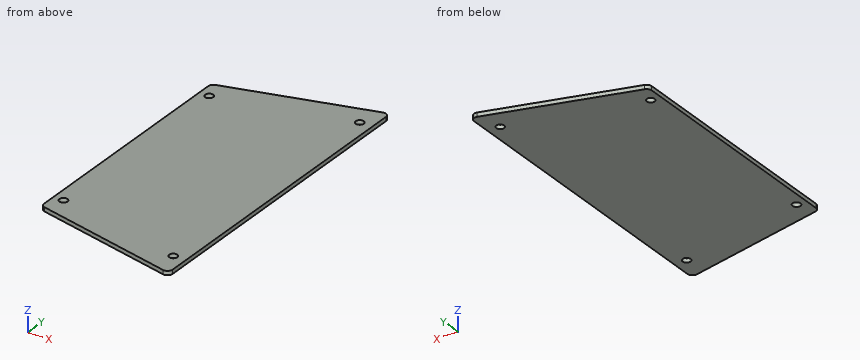
Autodesk Inventor part; units mm, degrees
ref_plane "YZ Plane" through (0, 0, 0) normal (1, 0, 0) x (0, 1, 0)
ref_plane "XZ Plane" through (0, 0, 0) normal (0, 1, 0) x (-1, 0, 0)
ref_plane "XY Plane" through (0, 0, 0) normal (0, 0, 1) x (1, 0, 0)
sketch "Esquisse1" plane through (0, 0, 0) normal (0, 0, 1) x (1, 0, 0)
  line L0 (0, 0) -> (60, 0)
  line L1 (60, 0) -> (60, 130)
  line L2 (60, 130) -> (0, 130)
  line L3 (0, 130) -> (0, 0)
  dimension "d0" = 130
  dimension "d1" = 60
extrude "Extrusion1" add sketch "Esquisse1" along normal blind 1.6
chamfer "Chanfrein1" distance 58 distance2 15 1 edges at (0, 130, 0.8) measured on face at (40, 130, 0.5333)
chamfer "Chanfrein2" distance 15 distance2 58 1 edges at (0, 0, 0.8) measured on face at (0, 76.6667, 1.0667)
fillet "Congé1" radius 2 6 edges at (60, 0, 0.8) (0, 15, 0.8) (0, 115, 0.8) (60, 130, 0.8) (58, 130, 0.8) (58, 0, 0.8)
sketch "Esquisse2" plane through (0, 0, 1.6) normal (0, 0, 1) x (1, 0, 0)
  circle A0 centre (4, 22) radius 1.6
  circle A1 centre (55, 10) radius 1.6
  circle A2 centre (4, 108) radius 1.6
  circle A3 centre (55, 120) radius 1.6
  line L0 (0, 113.4514) -> (0, 16.5486)
  arc A4 (57.4992, 0.1295) -> (60, 2.0658) centre (58, 2.0658) ccw
  arc A5 (60, 127.9342) -> (57.4992, 129.8705) centre (58, 127.9342) ccw
  point P0 (0, 0)
  dimension "d11" = 51
  dimension "d12" = 4
  dimension "d13" = 86
  dimension "d14" = 96.9029
  dimension "d15" = 5.4514
  dimension "d16" = 110
  dimension "d17" = 125.8684
  dimension "d18" = 7.9342
  dimension "d19" = 3.2
extrude "Extrusion2" cut sketch "Esquisse2" against normal through all
equation "\"d15\" = -0.5 * d13 + 0.5 * d14"
equation "\"d18\" = -0.5 * d16 + 0.5 * d17"
properties part number "PCBCapteurs" material "Résine phénolique"
Design review of the part built by this model. Coordinates are the model's own, in mm. Give positions to 0.01 mm unless a question says otherwise; leave off trailing zeros. Order: outer loops, then holes, each group sorted by start corner. A loop starts at its lowest first (then second) coordinate and runs counter-clockwise, first axis right, second up. Notation, with made-up numbers: (85, -24.75) -> (108, -24.75) arc R13 ccw to (108, -3.75) -> close; hole circle Ø2 at (-39, -12). An arc over 180 degrees is marked (long way). Write each question's results on one line, items separated by ' | '. Start each with the question number.
Q1. Add section B-B on x = 55. Give the boundary of the cut face in (y, z), and give its area (3 significant figures).
Q2. Add section C-C on z = 0.5. State how many separate pieces and enclosed holes the cut face has, and give its area (3 significant figures).
Q3. Wall thickness on L1, parallel to Y at x = 55, z = 0.9; L2, parallel to Y at x = 4, z = 0.55; L3, parallel to X at y = 21, z = 1.1: over which ranges is each line inside the solid? List them lowest first. Write a range as from..to.
Q4. Add section D-D on x = 4. Give the boundary of the cut face in (y, z).
Q5. Add section A-A on y = 22. Give the boundary of the cut face in (x, z), and give its area (3 significant figures).
Found:
1) outline: (0.78, 0) -> (8.4, 0) -> (8.4, 1.6) -> (0.78, 1.6) -> close; (11.6, 0) -> (118.4, 0) -> (118.4, 1.6) -> (11.6, 1.6) -> close; (121.6, 0) -> (129.22, 0) -> (129.22, 1.6) -> (121.6, 1.6) -> close | area: 195 mm2
2) separate pieces: 1 | enclosed holes: 4 | area: 6,890 mm2
3) L1: y = 0.78..8.4, 11.6..118.4, 121.6..129.22 | L2: y = 13.97..20.4, 23.6..106.4, 109.6..116.03 | L3: x = 0..2.75, 5.25..60
4) outline: (13.97, 0) -> (20.4, 0) -> (20.4, 1.6) -> (13.97, 1.6) -> close; (23.6, 0) -> (106.4, 0) -> (106.4, 1.6) -> (23.6, 1.6) -> close; (109.6, 0) -> (116.03, 0) -> (116.03, 1.6) -> (109.6, 1.6) -> close
5) outline: (0, 0) -> (2.4, 0) -> (2.4, 1.6) -> (0, 1.6) -> close; (5.6, 0) -> (60, 0) -> (60, 1.6) -> (5.6, 1.6) -> close | area: 90.9 mm2
